Verification items for this drawing (mm, ordinates from the low corner). A direction names the side the tool comes from. Round coordinates to 2 decimals unless told otherwise and drop trailing zeros. Write each loop counter-clockwise with the first axis right and the second up, starting at its lowest first coordinate (ties: lowest second). Pieces come first, ordered by that corner, then holes. Notation, with made-up numbers: M 1,27 L 42,27 A23 cw 42,58 Z; hole C -12.75,-10.5 d11. An arc over 180 degrees is marked long. Write each question's results on one line, items separated by ' | '.
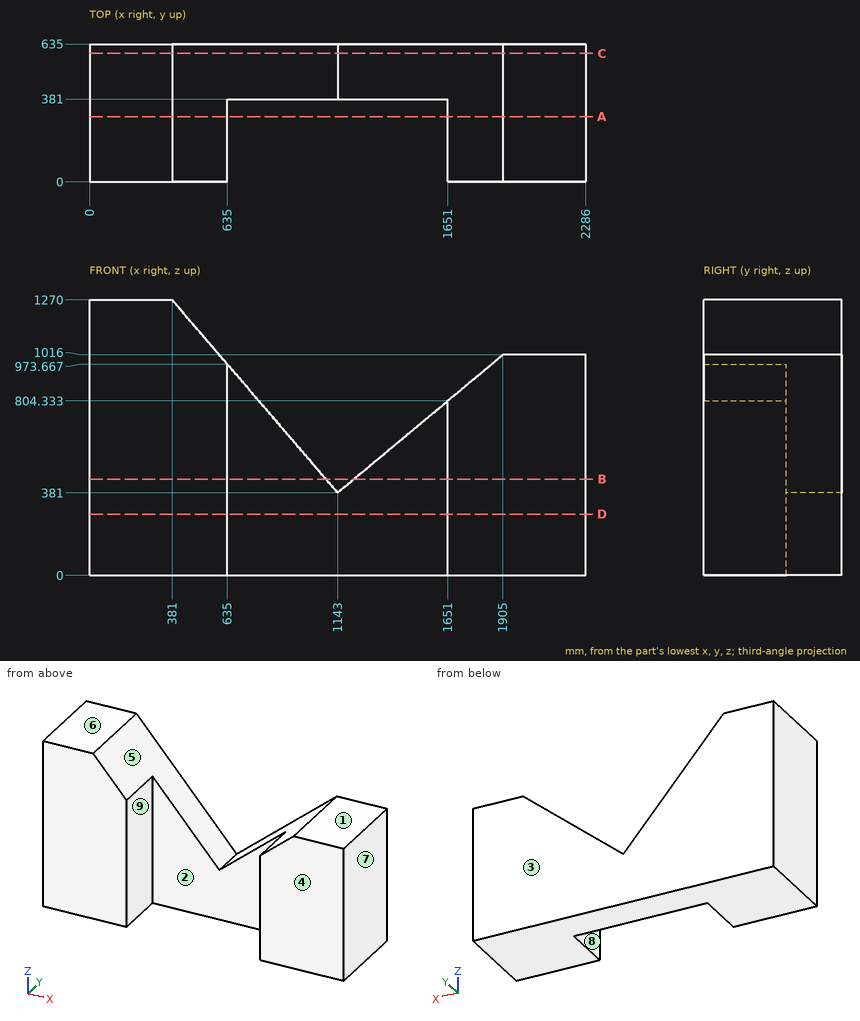
1) Sectioned sample at C-C, the plane y = 591.5. Record the cut outline in (x, z).
Calculated:
outline: M 0,0 L 2286,0 L 2286,1016 L 1905,1016 L 1143,381 L 381,1270 L 0,1270 Z
2) Sectioned sample at A-A, the plane y = 300. Record the cut outline in (x, z).
Calculated:
outline: M 0,0 L 635,0 L 635,973.67 L 381,1270 L 0,1270 Z; M 1651,0 L 2286,0 L 2286,1016 L 1905,1016 L 1651,804.33 Z
3) Sectioned sample at D-D, the plane z = 283. Record the cut outline in (x, y).
Calculated:
outline: M 0,0 L 635,0 L 635,381 L 1651,381 L 1651,0 L 2286,0 L 2286,635 L 0,635 Z
4) Sectioned sample at B-B, the plane z = 444. Record the cut outline in (x, y), and give its area (3 significant figures).
Calculated:
outline: M 0,0 L 635,0 L 635,381 L 1089,381 L 1089,635 L 0,635 Z; M 1218.6,381 L 1651,381 L 1651,0 L 2286,0 L 2286,635 L 1218.6,635 Z | area: 1,030,000 mm²
5) Material ranges on line 1 (X direction, y = 240.5, z = 91.5); line 2 (Z direction, x = 2144, y = 203); line 3 (X direction, y = 263, z = 885), recorded low to high. Write a range as [from, to].
Calculated:
line 1: x = [0, 635], [1651, 2286] | line 2: z = [0, 1016] | line 3: x = [0, 635], [1747.8, 2286]
6) Access from +Z, -Z, +X, -X, +Y, -Y to the whole of each face (thin tool, end or side, straight path). Record for the marked faces 1, 2, 3, 4 and 5.
Calculated:
face 1: +Z, +X, +Y, -Y | face 2: +Z, -Z, -Y | face 3: +Z, -Z, +X, -X, +Y | face 4: +Z, -Z, +X, -X, -Y | face 5: +Z, +Y, -Y
7) Draft check along X on the marked faces 6, 7, 8 and 9. Enter one of: pulls with the +X half, pulls with the -X half, needs draft (parallel to the pull), parting line crosses it, or undercut.
Calculated:
face 6: needs draft | face 7: pulls with the +X half | face 8: undercut | face 9: undercut
8) Depth check by flat-ended pin: P1, Ø1, axis at x = 745, z = 196, coming from the -Y side. Enter the tip coordinate at first touch or a pass-through.
Calculated:
P1: stops at y = 381
